Check sheet for the drawn part. Datum: minimum x, y, z corner. Units: mm. Round coordinates to 2 decimals unless told otherwise and drop trailing zeros. Write each loop counter-clockwise with the first axis right and the second up, starting at its lowest first coordinate (ties: lowest second). Pieces come first, ordered by that corner, then holes. Notation, with made-up numbers: (17, -35) - (66, -35) arc R21 cw to (66, -28) - close; hole circle Ø1 at (83, 87). An arc over 180 degrees is marked (long way). Answer as a JSON object with one key per item and string values.
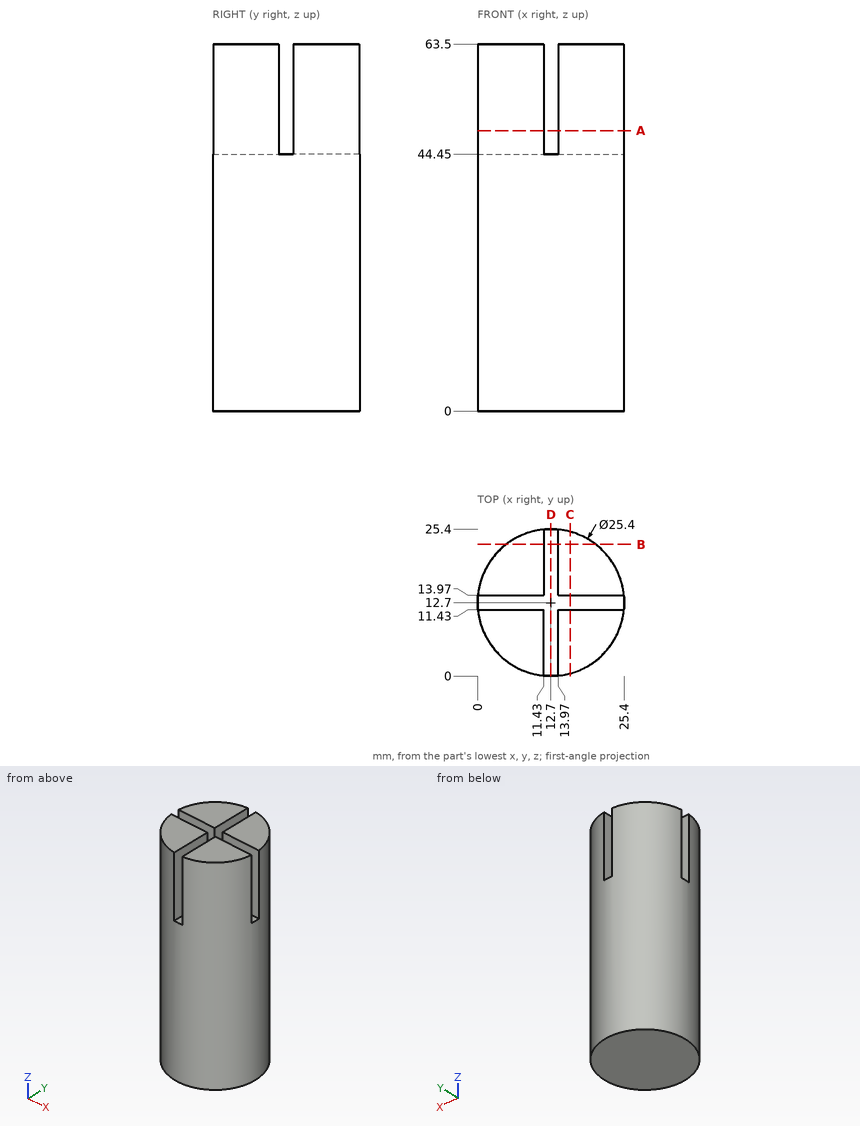
Q1. Section check A-A, the plane z = 48.5. Record the cut outline in (x, y), then the cut area to 3 significant figures.
Geometry check:
{"outline": "(0.06, 11.43) arc R12.7 ccw to (11.43, 0.06) - (11.43, 11.43) - close; (0.06, 13.97) - (11.43, 13.97) - (11.43, 25.34) arc R12.7 ccw to start; (13.97, 0.06) arc R12.7 ccw to (25.34, 11.43) - (13.97, 11.43) - close; (13.97, 13.97) - (25.34, 13.97) arc R12.7 ccw to (13.97, 25.34) - close", "area": "384 mm2"}
Q2. Gauge pin test, flat ends, axial feed: P1, Ø3, axis at x = 14.5, z = 57, coming from the -Y side; P2, Ø8, axis at y = 6.5, z = 33.5, coming from the -X side; P3, Ø9, axis at y = 6.5, z = 52, coming from the -X side. Record the tip position at first contact, or that the pin passes through.
Geometry check:
{"P1": "stops at y = 0.06", "P2": "stops at x = 0.19", "P3": "stops at x = 0.11"}
Q3. Material ranges on line 1 along Z through (x, y) = (11.5, 14.5); line 2 along Y through (x, z) = (16.75, 59.5); line 3 along Y through (x, z) = (12.25, 4), recorded low to high. Write a range as [from, to].
Geometry check:
{"line 1": "z = [0, 44.45]", "line 2": "y = [0.66, 11.43], [13.97, 24.74]", "line 3": "y = [0.01, 25.39]"}
Q4. Section check B-B, the plane y = 22.75. Record the cut outline in (x, z).
Geometry check:
{"outline": "(4.94, 0) - (20.46, 0) - (20.46, 63.5) - (13.97, 63.5) - (13.97, 44.45) - (11.43, 44.45) - (11.43, 63.5) - (4.94, 63.5) - close"}
Q5. Section check D-D, the plane x = 12.7. Record the cut outline in (y, z), then the cut area to 3 significant figures.
Geometry check:
{"outline": "(0, 0) - (25.4, 0) - (25.4, 44.45) - (0, 44.45) - close", "area": "1,130 mm2"}
Q6. Section check C-C, the plane x = 16. Record the cut outline in (y, z), then the cut area to 3 significant figures.
Geometry check:
{"outline": "(0.44, 0) - (24.96, 0) - (24.96, 63.5) - (13.97, 63.5) - (13.97, 44.45) - (11.43, 44.45) - (11.43, 63.5) - (0.44, 63.5) - close", "area": "1,510 mm2"}
